Part model, mm, in its own coordinate system. A direction names the side the tool comes from. Coordinates: 2 decimals unless noted, no trailing zeros. Loops run counter-clockwise (first coordinate to the right, second up) from the corner with the lowest first, then second, coordinate; pieces in that order, holes last. Notation, with made-up numbers: (78.25, -24.75) - (92.25, -24.75) arc R9 cw to (92.25, -7.75) - close; hole circle Ø1 at (-26.75, 88). An arc over 180 degrees is marked (long way). Use a Markdown table: item, result. Add a question column.
1) Band-saw the part on C-C (z = -172). Give the cut face in (x, y), plus the area to 3 significant figures.
2) Band-saw the part on A-A (z = -94). Give the number of separate pieces and of enclosed holes in the cut face, plus the area to 3 significant figures.
3) Pull direction X, two halves, no side cores. Call faces 4 (the face through (1, 430, 10)), 5 (the face through (1, 200, 1)), 6 (the face through (-126, 229, 16)): +X half, -X half, draft (parallel to the pull), parting line (faces both ways), or undercut.
4) Band-saw the part on B-B (y = 36.5). Give the cut face in (x, z).
5) Probe probe 1 along Y at (x, z) = (113.5, -141); probe 2 along Z at (x, y) = (108, 366); probe 3 along X at (y, z) = (357, 170). List the from-to ranges inside material, lowest first. Write a range as [from, to].
6) Tool access for faces 1 (the face through (-1, 230, 117.5)), 2 (the face through (-1, 240, -195)), 3 (the face through (1, 180, 1)): list every direction of +Z, -Z, +X, -X, +Y, -Y with a clear straight run to the whole face (end or side of a thin tool).
from build123d import *

# Parameters (mm, degrees)
SKETCH1_W           = 252
SKETCH1_H           = 410
SKETCH1_W_2         = 212
SKETCH1_H_2         = 370
BOSS_EXTRUDE1_DEPTH = 20
SKETCH2_W           = 20
SKETCH2_H           = 40
BOSS_EXTRUDE2_DEPTH = 460
BOSS_EXTRUDE3_START = 460
SKETCH1_3_W         = 252
SKETCH1_3_H         = 410
SKETCH1_3_W_2       = 212
SKETCH1_3_H_2       = 370
BOSS_EXTRUDE3_DEPTH = 20
SKETCH3_W           = 212
SKETCH3_H           = 40
BOSS_EXTRUDE4_DEPTH = 20
SKETCH4_W           = 20
SKETCH4_H           = 20
BOSS_EXTRUDE5_DEPTH = 330
SKETCH6_W           = 20
SKETCH6_H           = 20
BOSS_EXTRUDE6_DEPTH = 212
LPATTERN2_COUNT     = 2
LPATTERN2_PITCH     = 240
LPATTERN1_COUNT     = 2
LPATTERN1_PITCH     = 240
LPATTERN3_COUNT     = 2
LPATTERN3_PITCH     = 240


with BuildPart() as part:
    # Sketch1 → Boss-Extrude1 (new body)
    with BuildSketch(Plane(origin=(0, 0, 0), x_dir=(1, 0, 0), z_dir=(0, 1, 0))):
        Rectangle(SKETCH1_W, SKETCH1_H)
        Rectangle(SKETCH1_W_2, SKETCH1_H_2, mode=Mode.SUBTRACT)
    boss_extrude1 = extrude(amount=-BOSS_EXTRUDE1_DEPTH)

    # Sketch2 → Boss-Extrude2 (add)
    with BuildSketch(Plane(origin=(0, 0, 0), x_dir=(1, 0, 0), z_dir=(0, 1, 0))):
        with Locations((-116, 185)):
            Rectangle(SKETCH2_W, SKETCH2_H)
        with Locations((-116, -185)):
            Rectangle(SKETCH2_W, SKETCH2_H)
        with Locations((116, -185)):
            Rectangle(SKETCH2_W, SKETCH2_H)
        with Locations((116, 185)):
            Rectangle(SKETCH2_W, SKETCH2_H)
    extrude(amount=BOSS_EXTRUDE2_DEPTH)

    # Sketch1<3> → Boss-Extrude3 (add)
    with BuildSketch(Plane(origin=(0, 0, 0), x_dir=(1, 0, 0), z_dir=(0, 1, 0)).offset(BOSS_EXTRUDE3_START)):
        Rectangle(SKETCH1_3_W, SKETCH1_3_H)
        Rectangle(SKETCH1_3_W_2, SKETCH1_3_H_2, mode=Mode.SUBTRACT)
    extrude(amount=BOSS_EXTRUDE3_DEPTH)

    # Sketch3 → Boss-Extrude4 (add)
    with BuildSketch(Plane(origin=(0, 0, 0), x_dir=(1, 0, 0), z_dir=(0, 1, 0))):
        with Locations((0, -97.5)):
            Rectangle(SKETCH3_W, SKETCH3_H)
        with Locations((0, 97.5)):
            Rectangle(SKETCH3_W, SKETCH3_H)
    boss_extrude4 = extrude(amount=-BOSS_EXTRUDE4_DEPTH)

    # Sketch4 → Boss-Extrude5 (add)
    with BuildSketch(Plane(origin=(0, 0, 165), x_dir=(-1, 0, 0), z_dir=(0, 0, -1))):
        with Locations((-116, 190)):
            Rectangle(SKETCH4_W, SKETCH4_H)
        with Locations((116, 190)):
            Rectangle(SKETCH4_W, SKETCH4_H)
    boss_extrude5 = extrude(amount=BOSS_EXTRUDE5_DEPTH)

    # Sketch6 → Boss-Extrude6 (add)
    with BuildSketch(Plane.ZY.offset(-106)):
        with Locations((-195, 190)):
            Rectangle(SKETCH6_W, SKETCH6_H)
        with Locations((0, 190)):
            Rectangle(SKETCH6_W, SKETCH6_H)
        with Locations((195, 190)):
            Rectangle(SKETCH6_W, SKETCH6_H)
    boss_extrude6 = extrude(amount=BOSS_EXTRUDE6_DEPTH)

    # LPattern2: Boss-Extrude5 ×2
    with Locations(*[(0, i * LPATTERN2_PITCH, 0) for i in range(1, LPATTERN2_COUNT)]):
        add(boss_extrude5)

    # LPattern1: Boss-Extrude6 ×2
    with Locations(*[(0, i * LPATTERN1_PITCH, 0) for i in range(1, LPATTERN1_COUNT)]):
        add(boss_extrude6)

    # LPattern3: Boss-Extrude1, Boss-Extrude4 ×2
    with Locations(*[(0, i * LPATTERN3_PITCH, 0) for i in range(1, LPATTERN3_COUNT)]):
        add(boss_extrude1)
        add(boss_extrude4)


solid = part.part
Answer block:
| question | item | result |
|---|---|---|
| 1 | outline | (-126, -20) - (-106, -20) - (-106, 480) - (-126, 480) - close; (106, -20) - (126, -20) - (126, 480) - (106, 480) - close |
| 1 | area | 20,000 mm2 |
| 2 | separate pieces | 8 |
| 2 | enclosed holes | 0 |
| 2 | area | 12,500 mm2 |
| 3 | face 4 | undercut |
| 3 | face 5 | draft |
| 3 | face 6 | -X half |
| 4 | outline | (-126, -205) - (-106, -205) - (-106, -165) - (-126, -165) - close; (-126, 165) - (-106, 165) - (-106, 205) - (-126, 205) - close; (106, -205) - (126, -205) - (126, -165) - (106, -165) - close; (106, 165) - (126, 165) - (126, 205) - (106, 205) - close |
| 5 | probe 1 | [-20, 0], [180, 200], [220, 240], [420, 440], [460, 480] |
| 5 | probe 2 | [-205, -165], [165, 205] |
| 5 | probe 3 | [-126, -106], [106, 126] |
| 6 | face 1 | +Y, -Y |
| 6 | face 2 | +Z, -Z |
| 6 | face 3 | +X, -X |
